Part model, mm, in its own coordinate system. Give positions to 0.01 mm unless a question says otherwise; leave off trailing zeros. Write each loop counter-clockwise with the first axis right and the second up, starting at its lowest first coordinate (ties: lowest second). Pieces come first, ordered by that corner, then holes. Notation, with made-up numbers: M 12.5,62.5 L 69.5,62.5 A13 cw 69.5,66.5 Z; hole C 76.5,-30 d9. An arc over 180 degrees is marked long. Use a Markdown table: item, result. Add a question column.
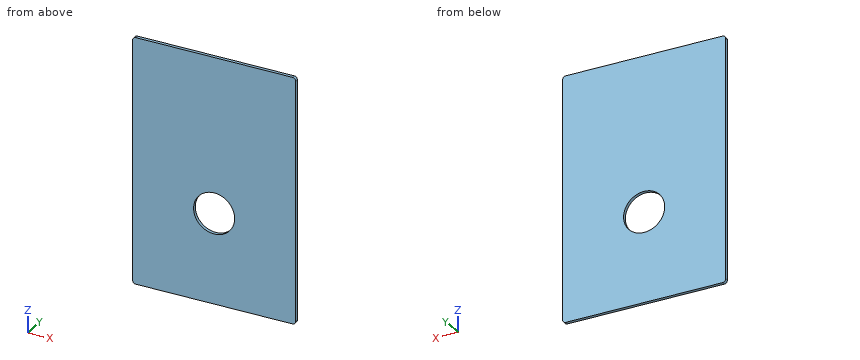
from build123d import *

# Parameters (mm, degrees)
SKETCH1_W           = 500
SKETCH1_H           = 755
BOSS_EXTRUDE1_DEPTH = 10
SKETCH3_R           = 63
CUT_EXTRUDE10_DEPTH = 11
FILLET1_R           = 10


with BuildPart() as part:
    # Sketch1 → Boss-Extrude1 (new body)
    with BuildSketch(Plane(origin=(0, 0, 0), x_dir=(1, 0, 0), z_dir=(0, 1, 0))):
        Rectangle(SKETCH1_W, SKETCH1_H)
    extrude(amount=BOSS_EXTRUDE1_DEPTH)

    # Sketch3 → Cut-Extrude10 (cut, through all)
    with BuildSketch(Plane(origin=(0, 0, 0), x_dir=(1, 0, 0), z_dir=(0, 1, 0))):
        with Locations((0, 100)):
            Circle(SKETCH3_R)
    extrude(amount=CUT_EXTRUDE10_DEPTH, mode=Mode.SUBTRACT)

    # Fillet1
    fillet1_edges = [part.edges().sort_by_distance(p)[0] for p in [
        (-250, 5, 377.5),
        (-250, 5, -377.5),
        (250, 5, -377.5),
        (250, 5, 377.5),
    ]]
    fillet(fillet1_edges, radius=FILLET1_R)


solid = part.part
1. Cut at A-A (x = 0). Write the cut outline in (y, z).
2. Cut at C-C (y = 6.5). Write the cut outline in (x, z).
3. Cut at B-B (z = -65). Write the cut outline in (x, y).
4. Drill centre lines: probe 1 along Z at (x, y) = (-4.5, 7.75); probe 2 along X at (y, z) = (4.75, -100); probe 3 along Z at (x, y) = (0, 5.5). Where is each one in solid material? Low to high. Write a range as [from, to].
A:
| question | item | result |
|---|---|---|
| 1 | outline | M 0,-377.5 L 10,-377.5 L 10,-163 L 0,-163 Z; M 0,-37 L 10,-37 L 10,377.5 L 0,377.5 Z |
| 2 | outline | M -250,-367.5 A10 ccw -240,-377.5 L 240,-377.5 A10 ccw 250,-367.5 L 250,367.5 A10 ccw 240,377.5 L -240,377.5 A10 ccw -250,367.5 Z; hole C 0,-100 d126 |
| 3 | outline | M -250,0 L -52.38,0 L -52.38,10 L -250,10 Z; M 52.38,0 L 250,0 L 250,10 L 52.38,10 Z |
| 4 | probe 1 | z = [-377.5, -162.84], [-37.16, 377.5] |
| 4 | probe 2 | x = [-250, -63], [63, 250] |
| 4 | probe 3 | z = [-377.5, -163], [-37, 377.5] |
